Here's how the part is built. I have some questions about the finished solid (model axes, mm). A direction names the side the tool comes from. Round coordinates to 2 decimals unless told otherwise and drop trailing zeros. Loops run counter-clockwise (first coordinate to the right, second up) from the corner with the lowest first, then second, coordinate; pieces in that order, holes last. Notation, with made-up numbers: M 32.25,79.25 L 58.25,79.25 A14 ccw 58.25,94.25 Z; hole C 36.5,19.5 d2. An arc over 180 degrees is marked long. Answer as CSV lines item,"result".
```python
from build123d import *

# Parameters (mm, degrees)
SKETCH_1_W          = 30
SKETCH_1_H          = 30
EXTRUDE_1_DEPTH     = 5
SKETCH_2_W          = 15
SKETCH_2_H          = 15
EXTRUDE_2_DEPTH     = 5
SKETCH_3_R          = 0.5
SKETCH_3_W          = 10.1
SKETCH_3_H          = 10.1
SKETCH_3_R_2        = 1.5
CUT_EXTRUDE_1_DEPTH = 10
SKETCH_4_R          = 3
CUT_EXTRUDE_2_DEPTH = 2


with BuildPart() as part:
    # 草图1 → 凸台-拉伸1 (new body)
    with BuildSketch(Plane(origin=(0, 0, 0), x_dir=(1, 0, 0), z_dir=(0, 1, 0))):
        Rectangle(SKETCH_1_W, SKETCH_1_H)
    extrude(amount=EXTRUDE_1_DEPTH)

    # 草图2 → 凸台-拉伸2 (add)
    with BuildSketch(Plane(origin=(0, 5, 0), x_dir=(1, 0, 0), z_dir=(0, 1, 0))):
        Rectangle(SKETCH_2_W, SKETCH_2_H)
    extrude(amount=EXTRUDE_2_DEPTH)

    # 草图3 → 切除-拉伸1 (cut)
    with BuildSketch(Plane(origin=(0, 10, 0), x_dir=(1, 0, 0), z_dir=(0, 1, 0))):
        with Locations((5.05, -5.05)):
            Circle(SKETCH_3_R)
        with Locations((5.05, 5.05)):
            Circle(SKETCH_3_R)
        with Locations((-5.05, 5.05)):
            Circle(SKETCH_3_R)
        with Locations((-5.05, -5.05)):
            Circle(SKETCH_3_R)
        Rectangle(SKETCH_3_W, SKETCH_3_H)
        with BuildLine():
            ThreePointArc((5.55, 5.05), (5.05, 5.55), (4.55, 5.05))
            Line((4.55, 5.05), (5.05, 5.05))
            Line((5.05, 5.05), (5.05, 4.55))
            ThreePointArc((5.05, 4.55), (5.403553391, 4.696446609), (5.55, 5.05))
        make_face()
        with BuildLine():
            Line((5.05, 5.05), (4.55, 5.05))
            ThreePointArc((4.55, 5.05), (4.696446609, 4.696446609), (5.05, 4.55))
            Line((5.05, 4.55), (5.05, 5.05))
        make_face()
        with BuildLine():
            ThreePointArc((-4.55, -5.05), (-4.696446609, -4.696446609), (-5.05, -4.55))
            Line((-5.05, -4.55), (-5.05, -5.05))
            Line((-5.05, -5.05), (-4.55, -5.05))
        make_face()
        with BuildLine():
            Line((-5.05, -5.05), (-5.05, -4.55))
            ThreePointArc((-5.05, -4.55), (-5.403553391, -5.403553391), (-4.55, -5.05))
            Line((-4.55, -5.05), (-5.05, -5.05))
        make_face()
        with BuildLine():
            Line((-5.05, 4.55), (-5.05, 5.05))
            Line((-5.05, 5.05), (-4.55, 5.05))
            ThreePointArc((-4.55, 5.05), (-5.403553391, 5.403553391), (-5.05, 4.55))
        make_face()
        with BuildLine():
            Line((-4.55, 5.05), (-5.05, 5.05))
            Line((-5.05, 5.05), (-5.05, 4.55))
            ThreePointArc((-5.05, 4.55), (-4.696446609, 4.696446609), (-4.55, 5.05))
        make_face()
        with BuildLine():
            ThreePointArc((5.55, -5.05), (5.403553391, -4.696446609), (5.05, -4.55))
            Line((5.05, -4.55), (5.05, -5.05))
            Line((5.05, -5.05), (4.55, -5.05))
            ThreePointArc((4.55, -5.05), (5.05, -5.55), (5.55, -5.05))
        make_face()
        with BuildLine():
            Line((5.05, -5.05), (5.05, -4.55))
            ThreePointArc((5.05, -4.55), (4.696446609, -4.696446609), (4.55, -5.05))
            Line((4.55, -5.05), (5.05, -5.05))
        make_face()
        with Locations(Location((-11.25, 0, 0), (0, 0, 270))):
            Circle(SKETCH_3_R_2)
        with Locations(Location((0, 11.25, 0), (0, 0, 270))):
            Circle(SKETCH_3_R_2)
        with Locations(Location((11.25, 0, 0), (0, 0, 270))):
            Circle(SKETCH_3_R_2)
        with Locations(Location((0, -11.25, 0), (0, 0, 270))):
            Circle(SKETCH_3_R_2)
    extrude(amount=-CUT_EXTRUDE_1_DEPTH, mode=Mode.SUBTRACT)

    # 草图4 → 切除-拉伸2 (cut)
    with BuildSketch(Plane(origin=(0, 5, 0), x_dir=(1, 0, 0), z_dir=(0, 1, 0))):
        with Locations(Location((11.25, 0, 0), (0, 0, 270))):
            Circle(SKETCH_4_R)
        with Locations(Location((0, -11.25, 0), (0, 0, 270))):
            Circle(SKETCH_4_R)
        with Locations(Location((-11.25, 0, 0), (0, 0, 270))):
            Circle(SKETCH_4_R)
        with Locations(Location((0, 11.25, 0), (0, 0, 270))):
            Circle(SKETCH_4_R)
    extrude(amount=-CUT_EXTRUDE_2_DEPTH, mode=Mode.SUBTRACT)


solid = part.part
```
1. I want a section at D-D, the plane z = 0. Please give me the cut outline in (x, y), and give its area (3 significant figures).
Evaluation:
outline,"M -15,0 L -12.75,0 L -12.75,3 L -14.25,3 L -14.25,5 L -15,5 Z; M -9.75,0 L -5.05,0 L -5.05,10 L -7.5,10 L -7.5,5 L -8.25,5 L -8.25,3 L -9.75,3 Z; M 5.05,0 L 9.75,0 L 9.75,3 L 8.25,3 L 8.25,5 L 7.5,5 L 7.5,10 L 5.05,10 Z; M 12.75,0 L 15,0 L 15,5 L 14.25,5 L 14.25,3 L 12.75,3 Z"
area,"82.0 mm²"
2. I want a section at C-C, the plane y = 1.5. Please give me the cut outline in (x, z).
Evaluation:
outline,"M -15,-15 L 15,-15 L 15,15 L -15,15 Z; hole C -11.25,0 d3; hole M -5.05,-4.55 A0.5 ccw long -4.55,-5.05 L 4.55,-5.05 A0.5 ccw long 5.05,-4.55 L 5.05,4.55 A0.5 ccw long 4.55,5.05 L -4.55,5.05 A0.5 ccw long -5.05,4.55 Z; hole C 0,-11.25 d3; hole C 0,11.25 d3; hole C 11.25,0 d3"
3. For P1, Ø6.5, axis at x = 12.5, z = -0.5, coming from the +Y side; P2, Ø3.5, axis at x = -11.25, z = 0, coming from the +Y side; P3, Ø4, axis at x = 3.5, y = 7.5, coming from the -Z side, each with a flat end and sliding along its axis, tell me the tip position at first contact or that it passes through.
Evaluation:
P1,"stops at y = 5"
P2,"stops at y = 3"
P3,"stops at z = -7.5"
4. I want a section at B-B, the plane z = 3.5. Please give me the cut outline in (x, y).
Evaluation:
outline,"M -15,0 L -5.05,0 L -5.05,10 L -7.5,10 L -7.5,5 L -15,5 Z; M 5.05,0 L 15,0 L 15,5 L 7.5,5 L 7.5,10 L 5.05,10 Z"
5. If I drill on line 1 (X direction, y = 2.25, z = 0); line 2 (Z direction, x = 3, y = 6.75); line 3 (X direction, y = 0.8, z = -11.25), over which ranges is the centre line in solid material (lowest first)? Write a range as [from, to].
Evaluation:
line 1,"x = [-15, -12.75], [-9.75, -5.05], [5.05, 9.75], [12.75, 15]"
line 2,"z = [-7.5, -5.05], [5.05, 7.5]"
line 3,"x = [-15, -1.5], [1.5, 15]"
6. We'd pull the mould along X, two halves only. Please class faces 4 (the flat face through (0, 7, 7.5)), 5 (the flat face through (-7.5, 7, 0)), 6 (the cylindrical face through (0.132, 4.014, 8.253)): pulls with the +X half, pulls with the -X half, needs draft (parallel to the pull), parting line crosses it, or undercut.
Evaluation:
face 4,"needs draft"
face 5,"pulls with the -X half"
face 6,"undercut"
7. I want a section at A-A, the plane x = 3.75. Please give me the cut outline in (y, z), and give its area (3 significant figures).
Evaluation:
outline,"M 0,-15 L 5,-15 L 5,-7.5 L 10,-7.5 L 10,-5.05 L 0,-5.05 Z; M 0,5.05 L 10,5.05 L 10,7.5 L 5,7.5 L 5,15 L 0,15 Z"
area,"124 mm²"
8. Which directions (+Z, -Z, +X, -X, +Y, -Y) give clear straight access to the entire face, cutting with the end or side of a thin tool? Please do faces 1 (the flat face through (7.5, 7, 0)), 2 (the flat face through (-1, 3, -13)), 3 (the flat face through (0, 5, -5.05)).
Evaluation:
face 1,"+Z, -Z, +X, +Y"
face 2,"+Y"
face 3,"+Y, -Y"
